Geometry: final body of the model. Coordinates: model frame, mm. Give positions to 0.01 mm unless a question says otherwise; leave off trailing zeros. Write each loop counter-clockwise with the first axis right and the second up, starting at its lowest first coordinate (ties: lowest second). Pieces come first, ordered by that corner, then holes.
```python
from build123d import *

# Parameters (mm, degrees)
F1_DEPTH = 63.5
F3_DEPTH = 51.8120278971
F4_R     = 3.4925
F5_DEPTH = 51.8120278971


with BuildPart() as f1:
    # F0 (on Right) → F1 (new body)
    with BuildSketch(Plane.YZ):
        Polygon((35.8086346566, 96.3798694051), (-25.6357367167, 0), (18.8142632833, 0), align=None)
    extrude(amount=F1_DEPTH)

    # F2 (on face) → F3 (cut, through all)
    with BuildSketch(Plane(origin=(0, -18.2274539145, 11.6204188118), x_dir=(1, 0, 0), z_dir=(0, -0.843218455, 0.5375710531))):
        Polygon((63.5, 100.5189700153), (31.75, 100.5189700153), (63.5, -13.7810299847), align=None)
        Polygon((0, 100.5189700153), (0, -13.7810299847), (31.75, 100.5189700153), align=None)
    extrude(amount=-F3_DEPTH, mode=Mode.SUBTRACT)

    # F4 (on face) → F5 (cut, through all)
    with BuildSketch(Plane(origin=(0, -18.2274539145, 11.6204188118), x_dir=(1, 0, 0), z_dir=(0, -0.843218455, 0.5375710531))):
        with Locations((31.75, 31.2540056114)):
            Circle(F4_R)
    extrude(amount=-F5_DEPTH, mode=Mode.SUBTRACT)


solid = f1.part
```
Item 1: Pin query (flat end, axial travel): pin 1 Ø5 at (x, z) = (33.5, 61) entering from -Y; pin 2 Ø1.5 at (x, z) = (32.5, 86) entering from +Y; pin 3 Ø3 at (x, y) = (38.5, -15) entering from +Z. Return the tip coordinate at first contact, or that it passes through.
Found:
pin 1: stops at y = 11.66
pin 2: stops at y = 34.11
pin 3: stops at z = 19.04
Item 2: Section B-B, the plane z = 16. Return the cut outline in (x, y).
Found:
outline: (5.27, -15.44) - (58.23, -15.44) - (52.69, 21.64) - (10.81, 21.64) - close
Item 3: Line query: L1, parallel to X at y = -1.5, z = 26; L2, parallel to Z at x = 15.5, y = -21; L3, parallel to Y at x = 26, z = 48. Output: solid intervals per line, ascending.
Found:
L1: x = 9.69 to 53.81
L2: z = 0 to 7.27
L3: y = 4.97 to 27.28
Item 4: Pull-direction query (Y, two-part tool) for faces 1 (the face through (31.306, -8.138, 27.447)), 2 (the face through (30.99, 9.29, 27.1)), 3 (the face through (50.93, 10.76, 30.46)); classes: +Y half, -Y half, draft (parallel to the pull), parting line (faces both ways), or undercut.
Found:
face 1: -Y half
face 2: undercut
face 3: +Y half
Item 5: Section A-A, the plane y = -12. Return the cut outline in (x, z).
Found:
outline: (2.04, 0) - (61.46, 0) - (56.45, 21.39) - (7.05, 21.39) - close
